Can you work these out from the model? Positions are in its coordinate system, mm. A direction names the side the tool comes from. Coordinates: 2 decimals unless noted, no trailing zeros. Order: outer loops, then holes, each group sorted by start corner. A loop starts at its lowest first (then second) coordinate and runs counter-clockwise, first axis right, second up. Notation, with made-up numbers: (13.25, 47.5) -> (46.25, 47.5) arc R18 cw to (46.25, 63.5) -> close; hole circle Ø9 at (30, -35.75). An arc over 180 degrees is marked (long way). Return JSON: item names as keys, results as strings. Group by question number.
1) For pin 1 (10 mm diameter, centred on x = 17, z = 410, fed in from -Y); pin 2 (6.5 mm diameter, centred on x = -5.5, z = 363, fed in from +Y); pin 3 (2 mm diameter, centred on y = -73.5, z = 407.5, fed in from -X); pin 4 (8 mm diameter, centred on x = 12.5, y = -47.5, fed in from -Z), each with a flat end and sliding along its axis, tell me the tip position at first contact or that it passes through.
2) For faces 4 (the flat face through (5, 8.89, 380)), 5 (the flat face through (7, -2.159, 380)), 6 (the flat face through (34, -125.302, 378)), 7 (the flat face through (-11, 2.794, 380)), which set-ups out of +Z, -Z, +X, -X, +Y, -Y let a thin tool reach every point of the face, with its end or its side?
3) Thinking about a two-plate mould opening in X: for faces 1 (the flat face through (-7.202, -28.509, 379.507)), 2 (the flat face through (0, -8.89, 380)), 3 (the flat face through (19.95, -17, 378)), which applies, +X half, -X half, draft (parallel to the pull), parting line (faces both ways), or undercut?
4) If we section it at B-B, the plane x = 7.5: Please give me the cut outline in (y, z).
5) If we section it at C-C, the plane y = -6: Please give me the cut outline in (x, z).
6) If I drill on probe 1 along Y at (x, z) = (0.5, 343); probe 2 along X at (y, z) = (-0.5, 373); probe 3 along Y at (x, z) = (9.5, 402), over which ranges is the centre line in solid material (lowest first)? Write a range as from..to.
7) If we section it at A-A, the plane x = 14: Please give me the cut outline in (y, z), then the cut area to 3 significant figures.
from build123d import *

# Parameters (mm, degrees)
BOSS_EXTRUDE1_DEPTH = 457.2
SKETCH2_W           = 42.050956734
SKETCH2_H           = 23.599286926
CUT_EXTRUDE1_DEPTH  = 800
SKETCH3_W           = 114.4
SKETCH3_H           = 56.436670765
BOSS_EXTRUDE2_DEPTH = 10
SKETCH4_W           = 114.4
SKETCH4_H           = 4.244670765
CUT_EXTRUDE2_DEPTH  = 10
SKETCH7_W           = 48.1
SKETCH7_H           = 52.192
CUT_EXTRUDE3_DEPTH  = 42
SKETCH8_W           = 0.9
SKETCH8_H           = 40
CUT_EXTRUDE4_DEPTH  = 90
BOSS_EXTRUDE3_DEPTH = 10


with BuildPart() as part:
    # Sketch1 → Boss-Extrude1 (new body, symmetric)
    with BuildSketch(Plane.XY):
        Polygon((-19.05, 8.89), (19.05, 8.89), (19.05, 2.794), (3.81, 2.794), (3.81, -2.159), (9.779, -2.159), (9.779, -2.8321), (4.695818344, -8.89), (-4.695818344, -8.89), (-9.779, -2.8321), (-9.779, -2.159), (-3.81, -2.159), (-3.81, 2.794), (-19.05, 2.794), align=None)
    boss_extrude1 = extrude(amount=BOSS_EXTRUDE1_DEPTH, both=True)

    # Sketch2 → Cut-Extrude1 (cut)
    with BuildSketch(Plane(origin=(0, 0, -457.2), x_dir=(-1, 0, 0), z_dir=(0, 0, -1))):
        Rectangle(SKETCH2_W, SKETCH2_H)
    cut_extrude1 = extrude(amount=-CUT_EXTRUDE1_DEPTH, mode=Mode.SUBTRACT)

    # Sketch3 → Boss-Extrude2 (add)
    with BuildSketch(Plane(origin=(19.05, 0, 0), x_dir=(0, 0, -1), z_dir=(1, 0, 0))):
        with Locations((-400, -19.328335383)):
            Rectangle(SKETCH3_W, SKETCH3_H)
    extrude(amount=BOSS_EXTRUDE2_DEPTH)

    # Mirror1: Boss-Extrude1, Cut-Extrude1 across plane
    add(boss_extrude1.mirror(Plane(origin=(0, -17.206, 0), x_dir=(0, 0, 1), z_dir=(0, -1, 0))))
    add(cut_extrude1.mirror(Plane(origin=(0, -17.206, 0), x_dir=(0, 0, 1), z_dir=(0, -1, 0))), mode=Mode.SUBTRACT)

    # Sketch4 → Cut-Extrude2 (cut)
    with BuildSketch(Plane.ZY.offset(-19.05)):
        with Locations((400, -45.424335383)):
            Rectangle(SKETCH4_W, SKETCH4_H)
    extrude(amount=-CUT_EXTRUDE2_DEPTH, mode=Mode.SUBTRACT)

    # Sketch7 → Cut-Extrude3 (cut)
    with BuildSketch(Plane.XY.offset(457.2)):
        with Locations((5, -17.206)):
            Rectangle(SKETCH7_W, SKETCH7_H)
    extrude(amount=-CUT_EXTRUDE3_DEPTH, mode=Mode.SUBTRACT)

    # Sketch8 → Cut-Extrude4 (cut)
    with BuildSketch(Plane(origin=(0, 0, 342.8), x_dir=(-1, 0, 0), z_dir=(0, 0, -1))):
        with Locations((-19.5, -17.206)):
            Rectangle(SKETCH8_W, SKETCH8_H)
    extrude(amount=-CUT_EXTRUDE4_DEPTH, mode=Mode.SUBTRACT)

    # Sketch10 → Boss-Extrude3 (add)
    with BuildSketch(Plane(origin=(29.05, 0, 0), x_dir=(0, 0, -1), z_dir=(1, 0, 0))):
        Polygon((-425.2, 18.89), (-332.8, 18.89), (-332.8, -53.302), (-332.8, -125.302), (-425.2, -125.302), (-425.2, -53.302), align=None)
    extrude(amount=BOSS_EXTRUDE3_DEPTH)


solid = part.part
Result sheet:
{
 "1": {"pin 1": "stops at y = -43.3", "pin 2": "stops at y = 8.89", "pin 3": "stops at x = 29.05", "pin 4": "passes through"},
 "2": {"face 4": "+Z, -Z, -X, +Y", "face 5": "+Z, -Z", "face 6": "+Z, -Z, +X, -X, -Y", "face 7": "+Z, -Z, -X"},
 "3": {"face 1": "-X half", "face 2": "draft", "face 3": "undercut"},
 "4": {"outline": "(-43.3, 342.8) -> (-37.21, 342.8) -> (-37.21, 415.2) -> (-43.3, 415.2) -> close; (-32.25, 342.8) -> (-28.86, 342.8) -> (-28.86, 415.2) -> (-32.25, 415.2) -> close; (-5.55, 342.8) -> (-2.16, 342.8) -> (-2.16, 415.2) -> (-5.55, 415.2) -> close; (2.79, 342.8) -> (8.89, 342.8) -> (8.89, 415.2) -> (2.79, 415.2) -> close"},
 "5": {"outline": "(-7.12, 342.8) -> (7.12, 342.8) -> (7.12, 415.2) -> (-7.12, 415.2) -> close; (19.95, 342.8) -> (29.05, 342.8) -> (29.05, 332.8) -> (39.05, 332.8) -> (39.05, 425.2) -> (29.05, 425.2) -> (29.05, 415.2) -> (19.95, 415.2) -> close"},
 "6": {"probe 1": "y = -43.3..-25.52, -8.89..8.89", "probe 2": "x = -3.81..3.81, 19.95..39.05", "probe 3": "y = -43.3..-37.21, -32.25..-31.25, -3.16..-2.16, 2.79..8.89"},
 "7": {"outline": "(-43.3, 342.8) -> (-37.21, 342.8) -> (-37.21, 415.2) -> (-43.3, 415.2) -> close; (2.79, 342.8) -> (8.89, 342.8) -> (8.89, 415.2) -> (2.79, 415.2) -> close", "area": "883 mm2"}
}
